The drawing under review shows one solid part. Ordinate dimensions are in mm from its lowest x, y, z. A direction names the side the tool comes from. Round coordinates to 2 decimals unless told otherwise and drop trailing zeros. Write each loop counter-clockwise with the first axis right and the second up, starting at its lowest first coordinate (ties: lowest second). Pieces come first, ordered by that corner, then holes.
Item 1: Add section B-B (x = 6). Give the boundary of the cut face in (y, z), plus the area to 3 significant figures.
Item 2: Add section D-D (z = 33.5). Give the boundary of the cut face in (x, y) (3 decimals), plus the area to 3 significant figures.
Item 3: Machinability: for the marked faces 1, 2 and 3, which of the approach directions +Z, -Z, +X, -X, +Y, -Y give a long, thin tool a straight path to every point of the face, cutting with its end or side? Answer none if there is none.
Item 4: Clearance check with flat-ended pins moving along their axes: pin 1 Ø10 at (y, z) = (33, 24.5) entering from +X; pin 2 Ø24 at (x, z) = (68.5, 20) entering from -Y; pin 3 Ø10 at (y, z) = (15, 9) entering from -X; pin 4 Ø3 at (x, z) = (29.5, 21) entering from -Y. State where each tip first meets the part, or that it passes through.
Item 5: To check wall thickness, follow L1, parallel to Y at x = 14.5, z = 32.5; L2, parallel to X at y = 43, z = 24; L3, parallel to Y at x = 58, z = 17. State the ranges of each line that lie inside material, in increasing order.
Item 6: Add section C-C (y = 18). Give the boundary of the cut face in (x, z), plus the area to 3 significant figures.
Item 7: Add section A-A (z = 28). Give the boundary of the cut face in (x, y).
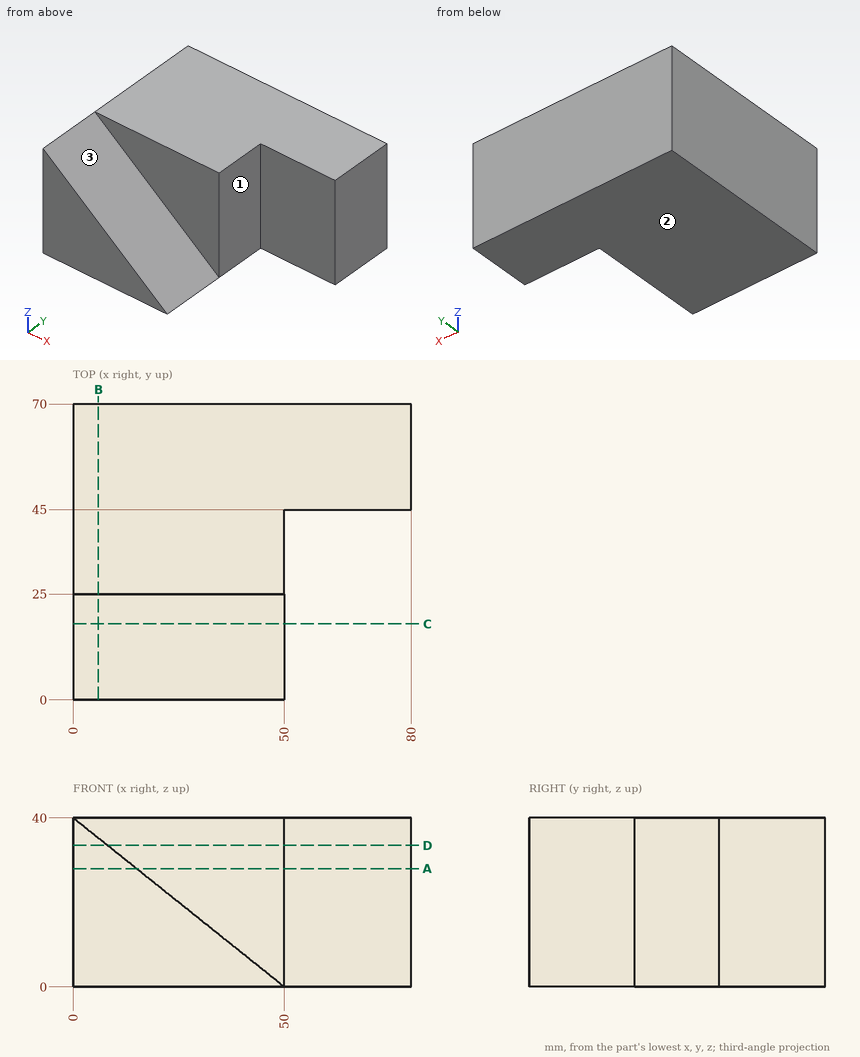
Numbers:
1. outline: (0, 0) - (70, 0) - (70, 40) - (25, 40) - (25, 35.2) - (0, 35.2) - close
1. area: 2,680 mm2
2. outline: (0, 0) - (8.125, 0) - (8.125, 25) - (50, 25) - (50, 45) - (80, 45) - (80, 70) - (0, 70) - close
2. area: 3,200 mm2
3. face 1: +Z, -Z, +X, -Y
3. face 2: -Z, +X, -X, +Y, -Y
3. face 3: +Z, +X, -Y
4. pin 1: stops at x = 50
4. pin 2: stops at y = 45
4. pin 3: stops at x = 0
4. pin 4: stops at y = 25
5. L1: y = 25 to 70
5. L2: x = 0 to 50
5. L3: y = 45 to 70
6. outline: (0, 0) - (50, 0) - (0, 40) - close
6. area: 1,000 mm2
7. outline: (0, 0) - (15, 0) - (15, 25) - (50, 25) - (50, 45) - (80, 45) - (80, 70) - (0, 70) - close
